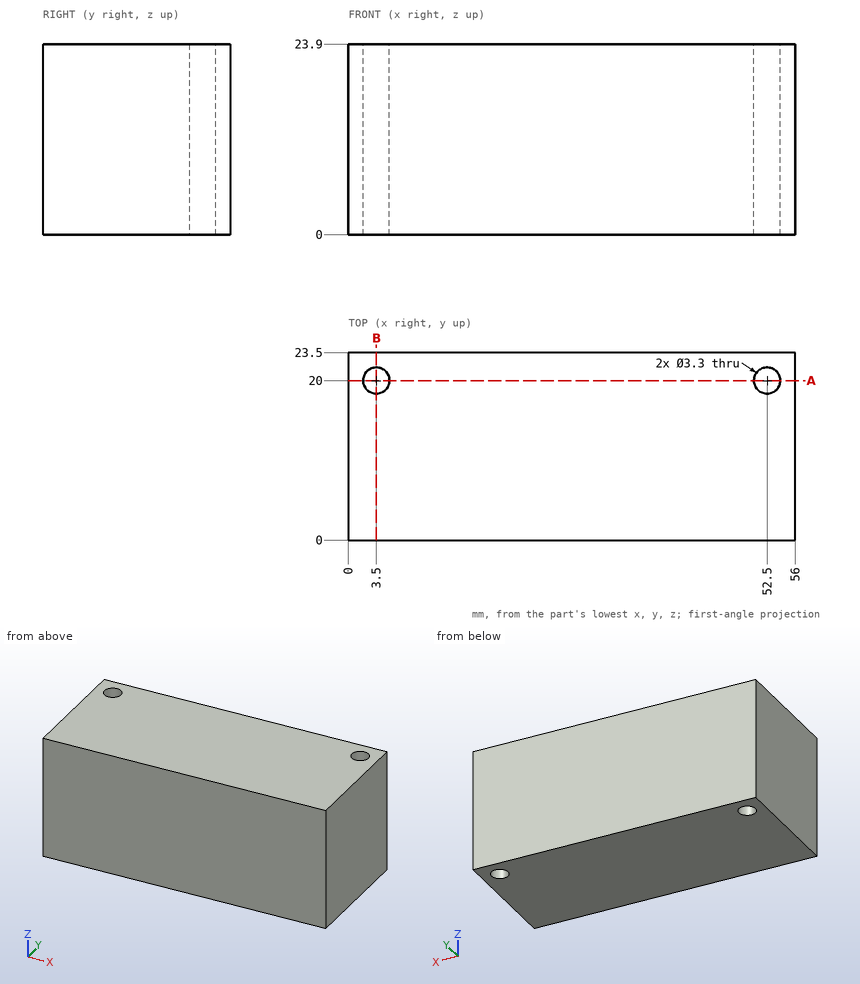
Source: three-view drawing plus pictorial views. Frame: mm from the lowest corner of the part. Coordinates: 2 decimals unless noted, no trailing zeros. Write each loop counter-clockwise with the first axis right and the second up, starting at its lowest first coordinate (ties: lowest second). Pieces come first, ordered by that corner, then holes. Notation, with made-up numbers: (64.5, 29) -> (81.5, 29) arc R16 ccw to (81.5, 49) -> close; hole circle Ø5 at (38, -18.75). An arc over 180 degrees is marked (long way). Write each question's results on one line, items separated by ' | '.
Item 1: Material intervals for probe 1 along X at (y, z) = (20, 11.75); probe 2 along Y at (x, z) = (3.5, 10), sorted ascending.
Conclusion:
probe 1: x = 0 to 1.85, 5.15 to 50.85, 54.15 to 56 | probe 2: y = 0 to 18.35, 21.65 to 23.5
Item 2: Section query B-B on x = 3.5. Return loops of the section in (y, z), plus the area to 3 significant figures.
Conclusion:
outline: (0, 0) -> (18.35, 0) -> (18.35, 23.9) -> (0, 23.9) -> close; (21.65, 0) -> (23.5, 0) -> (23.5, 23.9) -> (21.65, 23.9) -> close | area: 483 mm^2
Item 3: Section query A-A on y = 20. Return loops of the section in (x, z).
Conclusion:
outline: (0, 0) -> (1.85, 0) -> (1.85, 23.9) -> (0, 23.9) -> close; (5.15, 0) -> (50.85, 0) -> (50.85, 23.9) -> (5.15, 23.9) -> close; (54.15, 0) -> (56, 0) -> (56, 23.9) -> (54.15, 23.9) -> close
